Verification items for the finished model (mm, model axes). Face numbers are marked on the shaded views. A direction names the side the tool comes from. Round coordinates to 2 decimals unless told otherwise and drop trailing zeros. Loops run counter-clockwise (first coordinate to the right, second up) from the corner with the lowest first, then second, coordinate; pieces in that order, holes last. Notation, with made-up numbers: M -29.75,70.25 L -9.75,70.25 A22 cw -9.75,106.25 Z; hole C 4,12 d9. An arc over 180 degrees is marked long. One line per item, written item: value.
from build123d import *

# Parameters (mm, degrees)
BOX032_W          = 4
BOX032_H          = 6
BOX032_DEPTH      = 16
BOX033_W          = 4
BOX033_H          = 6
BOX033_DEPTH      = 16
CYLINDER022_R     = 7.5
CYLINDER022_DEPTH = 14
CYLINDER021_R     = 12
CYLINDER021_DEPTH = 14
FILLET005_R       = 1
FILLET006_R       = 1
CYLINDER009_R     = 1.5
CYLINDER009_DEPTH = 6
CYLINDER010_R     = 1.5
CYLINDER010_DEPTH = 6
CYLINDER011_R     = 1.5
CYLINDER011_DEPTH = 6
CYLINDER008_R     = 1.5
CYLINDER008_DEPTH = 6
BOX028_W          = 9
BOX028_H          = 3
BOX028_DEPTH      = 4
BOX029_W          = 9
BOX029_H          = 3
BOX029_DEPTH      = 4
BOX026_W          = 9
BOX026_H          = 3
BOX026_DEPTH      = 4
BOX027_W          = 9
BOX027_H          = 3
BOX027_DEPTH      = 4
BOX025_W          = 97
BOX025_H          = 32
BOX025_DEPTH      = 4
FILLET008_R       = 2


with BuildPart() as obj1:
    # Sphere → Sphere (revolve)
    with BuildSketch(Plane(origin=(39, 0, -12), x_dir=(1, 0, 0), z_dir=(0, -1, 0))):
        with BuildLine():
            ThreePointArc((0, -8), (8, 0), (0, 8))
            Line((0, 8), (0, -8))
        make_face()
    revolve(axis=Axis((39, 0, -12), (0, 0, 1)))


with BuildPart() as cubo026:
    # Box032 → Box032 (new body)
    with BuildSketch(Plane(origin=(37, -12, -19), x_dir=(1, 0, 0), z_dir=(0, 0, 1))):
        with Locations((2, 3)):
            Rectangle(BOX032_W, BOX032_H)
    extrude(amount=BOX032_DEPTH)


with BuildPart() as cubo027:
    # Box033 → Box033 (new body)
    with BuildSketch(Plane(origin=(37, 6, -19), x_dir=(1, 0, 0), z_dir=(0, 0, 1))):
        with Locations((2, 3)):
            Rectangle(BOX033_W, BOX033_H)
    extrude(amount=BOX033_DEPTH)


with BuildPart() as cilindro022:
    # Cylinder022 → Cylinder022 (new body)
    with BuildSketch(Plane(origin=(39, 0, -18), x_dir=(1, 0, 0), z_dir=(0, 0, 1))):
        Circle(CYLINDER022_R)
    extrude(amount=CYLINDER022_DEPTH)


with BuildPart() as fillet006:
    # Cylinder021 → Cylinder021 (new body)
    with BuildSketch(Plane(origin=(39, 0, -18), x_dir=(1, 0, 0), z_dir=(0, 0, 1))):
        Circle(CYLINDER021_R)
    extrude(amount=CYLINDER021_DEPTH)

    # Cut041: cut Cilindro022
    add(cilindro022.part, mode=Mode.SUBTRACT)

    # Cut042: cut Cubo027
    add(cubo027.part, mode=Mode.SUBTRACT)

    # Cut043: cut Cubo026
    add(cubo026.part, mode=Mode.SUBTRACT)

    # Cut044: cut obj1
    add(obj1.part, mode=Mode.SUBTRACT)

    # Fillet005
    fillet005_edges = [fillet006.edges().sort_by_distance(p)[0] for p in [
        (37, 9.530288, -18),
        (37, -9.530288, -18),
        (31.5, 0, -18),
    ]]
    fillet(fillet005_edges, radius=FILLET005_R)

    # Fillet006
    fillet006_edges = [fillet006.edges().sort_by_distance(p)[0] for p in [
        (41, 9.530288, -18),
        (44.968668, -4.541476, -18),
        (41, -9.530288, -18),
        (44.968668, 4.541476, -18),
    ]]
    fillet(fillet006_edges, radius=FILLET006_R)


with BuildPart() as obj2:
    # Sphere001 → Sphere001 (revolve)
    with BuildSketch(Plane(origin=(39, 0, -12), x_dir=(1, 0, 0), z_dir=(0, -1, 0))):
        with BuildLine():
            ThreePointArc((0, -8), (8, 0), (0, 8))
            Line((0, 8), (0, -8))
        make_face()
    revolve(axis=Axis((39, 0, -12), (0, 0, 1)))


with BuildPart() as cilindro009:
    # Cylinder009 → Cylinder009 (new body)
    with BuildSketch(Plane(origin=(25.6, -15.75, -4), x_dir=(1, 0, 0), z_dir=(0, 0, 1))):
        Circle(CYLINDER009_R)
    extrude(amount=CYLINDER009_DEPTH)


with BuildPart() as cilindro010:
    # Cylinder010 → Cylinder010 (new body)
    with BuildSketch(Plane(origin=(-25.8, -15.75, -4), x_dir=(1, 0, 0), z_dir=(0, 0, 1))):
        Circle(CYLINDER010_R)
    extrude(amount=CYLINDER010_DEPTH)


with BuildPart() as cilindro011:
    # Cylinder011 → Cylinder011 (new body)
    with BuildSketch(Plane(origin=(-25.8, 14.25, -4), x_dir=(1, 0, 0), z_dir=(0, 0, 1))):
        Circle(CYLINDER011_R)
    extrude(amount=CYLINDER011_DEPTH)


with BuildPart() as cilindro008:
    # Cylinder008 → Cylinder008 (new body)
    with BuildSketch(Plane(origin=(25.6, 14.25, -4), x_dir=(1, 0, 0), z_dir=(0, 0, 1))):
        Circle(CYLINDER008_R)
    extrude(amount=CYLINDER008_DEPTH)


with BuildPart() as cubo022:
    # Box028 → Box028 (new body)
    with BuildSketch(Plane(origin=(21, 15, -4), x_dir=(1, 0, 0), z_dir=(0, 0, 1))):
        with Locations((4.5, 1.5)):
            Rectangle(BOX028_W, BOX028_H)
    extrude(amount=BOX028_DEPTH)


with BuildPart() as cubo023:
    # Box029 → Box029 (new body)
    with BuildSketch(Plane(origin=(21, -20, -4), x_dir=(1, 0, 0), z_dir=(0, 0, 1))):
        with Locations((4.5, 1.5)):
            Rectangle(BOX029_W, BOX029_H)
    extrude(amount=BOX029_DEPTH)


with BuildPart() as cubo020:
    # Box026 → Box026 (new body)
    with BuildSketch(Plane(origin=(-30, 15, -4), x_dir=(1, 0, 0), z_dir=(0, 0, 1))):
        with Locations((4.5, 1.5)):
            Rectangle(BOX026_W, BOX026_H)
    extrude(amount=BOX026_DEPTH)


with BuildPart() as cubo021:
    # Box027 → Box027 (new body)
    with BuildSketch(Plane(origin=(-30, -20, -4), x_dir=(1, 0, 0), z_dir=(0, 0, 1))):
        with Locations((4.5, 1.5)):
            Rectangle(BOX027_W, BOX027_H)
    extrude(amount=BOX027_DEPTH)


with BuildPart() as obj3:
    # Box025 → Box025 (new body)
    with BuildSketch(Plane(origin=(-45, -17, -4), x_dir=(1, 0, 0), z_dir=(0, 0, 1))):
        with Locations((48.5, 16)):
            Rectangle(BOX025_W, BOX025_H)
    extrude(amount=BOX025_DEPTH)

    # Fusion008: union Cubo020, Cubo021
    add(cubo020.part)
    add(cubo021.part)

    # Fusion009: union Cubo022, Cubo023
    add(cubo022.part)
    add(cubo023.part)

    # Cut021: cut Cilindro008
    add(cilindro008.part, mode=Mode.SUBTRACT)

    # Cut022: cut Cilindro011
    add(cilindro011.part, mode=Mode.SUBTRACT)

    # Cut023: cut Cilindro010
    add(cilindro010.part, mode=Mode.SUBTRACT)

    # Cut024: cut Cilindro009
    add(cilindro009.part, mode=Mode.SUBTRACT)

    # Cut040: cut obj2
    add(obj2.part, mode=Mode.SUBTRACT)

    # Fusion010: union Fillet006
    add(fillet006.part)

    # Fillet008
    fillet008_edges = [obj3.edges().sort_by_distance(p)[0] for p in [
        (52, -17, -2),
        (52, 15, -2),
    ]]
    fillet(fillet008_edges, radius=FILLET008_R)


solid = obj3.part
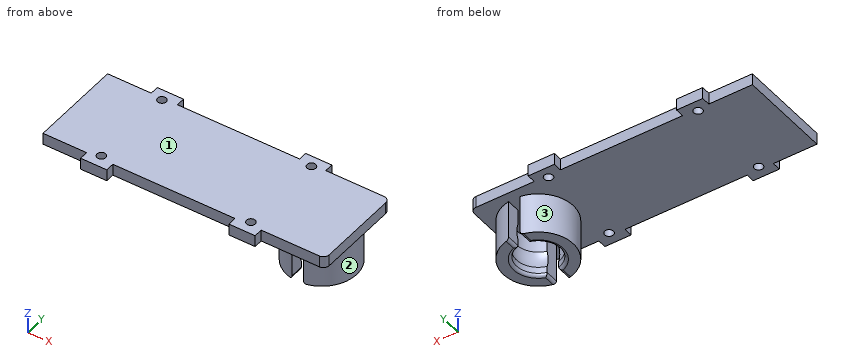
(1) Sectioned sample at A-A on x = -25.8. Enter the section's corners in (y, z).
Completed:
outline: M -20,-4 L -17.25,-4 L -17.25,0 L -20,0 Z; M -14.25,-4 L 12.75,-4 L 12.75,0 L -14.25,0 Z; M 15.75,-4 L 18,-4 L 18,0 L 15.75,0 Z
(2) Thickness scan on L1, parallel to Y at x = 25.6, z = -1.5; L2, parallel to X at y = 14.25, z = -1.45; L3, parallel to X at y = -15.75, z = -2.55. Record the ranges inside material, lowest first. Write a range as from..to.
Completed:
L1: y = -20..-17.25, -14.25..12.75, 15.75..18
L2: x = -45..-27.3, -24.3..24.1, 27.1..51.56
L3: x = -45..-27.3, -24.3..24.1, 27.1..51.85
(3) Tool access check on the marked faces 1, 2 and 3. Record the directions out of +Z, -Z, +X, -X, +Y, -Y that give a thin tool (end or side, any length) a straight path to the whole face; none if there is none.
Completed:
face 1: +Z, +X, -X, +Y, -Y
face 2: -Z, +X
face 3: -Z, -X
(4) Sectioned sample at B-B on z = -11.25. Enter the section's corners in (x, y).
Completed:
outline: M 37,-11.83 L 37,-7.71 A7.96 cw 37,7.71 L 37,11.83 A12 ccw Z; M 41,-11.83 A12 ccw 41,11.83 L 41,7.71 A7.96 cw 41,-7.71 Z
(5) Sectioned sample at C-C on z = -2. Enter the section's corners in (x, y).
Completed:
outline: M -45,-17 L -30,-17 L -30,-20 L -21,-20 L -21,-17 L 21,-17 L 21,-20 L 30,-20 L 30,-17 L 50,-17 A2 ccw 52,-15 L 52,13 A2 ccw 50,15 L 30,15 L 30,18 L 21,18 L 21,15 L -21,15 L -21,18 L -30,18 L -30,15 L -45,15 Z; hole C -25.8,-15.75 d3; hole C -25.8,14.25 d3; hole C 25.6,-15.75 d3; hole C 25.6,14.25 d3
(6) Sectioned sample at D-D on x = 28. Enter the section's corners in (y, z).
Completed:
outline: M -20,-4 L -4.8,-4 L -4.8,-18 L 4.8,-18 L 4.8,-4 L 18,-4 L 18,0 L -20,0 Z
(7) Depth check by flat-ended pin: pin 1 Ø8 at (x, y) = (-23, -11) entering from -Z; pin 2 Ø0.9 at (y, z) = (17, -2) entering from -X; pin 3 Ø3.5 at (y, z) = (10, -9) entering from -X. Enter the tip coordinate at first touch or a pass-through.
Completed:
pin 1: stops at z = -4
pin 2: stops at x = -30
pin 3: stops at x = 30.29
